```python
from build123d import *

# Parameters (mm, degrees)
BOSS_EXTRUDE1_DEPTH     = 76.2
SKETCH2_R               = 22.225
SKETCH2_R_2             = 4.7625
CUT_EXTRUDE2_DEPTH      = 34.20727615
CUT_EXTRUDE2_DEPTH_BACK = 31.29272385
CUT_EXTRUDE3_REACH      = 179.8
SKETCH3_R               = 6.35
SKETCH5_R               = 5.428392571
CUT_EXTRUDE4_DEPTH      = 76.2


with BuildPart() as part:
    # Sketch1 → Boss-Extrude1 (new body)
    with BuildSketch(Plane.XY):
        with BuildLine():
            Line((-88.9, -4.89272385), (73.025, -4.89272385))
            ThreePointArc((73.025, -4.89272385), (75.27006403, -5.82265982), (76.2, -8.06772385))
            Line((76.2, -8.06772385), (76.2, -30.29272385))
            Line((76.2, -30.29272385), (88.9, -30.29272385))
            Line((88.9, -30.29272385), (88.9, -4.89272385))
            Line((88.9, -4.89272385), (88.9, 7.80727615))
            Line((88.9, 7.80727615), (-73.025, 7.80727615))
            ThreePointArc((-73.025, 7.80727615), (-75.27006403, 8.73721212), (-76.2, 10.98227615))
            Line((-76.2, 10.98227615), (-76.2, 33.20727615))
            Line((-76.2, 33.20727615), (-88.9, 33.20727615))
            Line((-88.9, 33.20727615), (-88.9, 4.89272385))
            Line((-88.9, 4.89272385), (-88.9, -4.89272385))
        make_face()
    extrude(amount=BOSS_EXTRUDE1_DEPTH)

    # Sketch2 → Cut-Extrude2 (cut, two sides)
    with BuildSketch(Plane(origin=(0, 0, 0), x_dir=(1, 0, 0), z_dir=(0, 1, 0))) as cut_extrude2_sk:
        with Locations((0, -38.1)):
            Circle(SKETCH2_R)
        with Locations((-44.45, -38.1)):
            Circle(SKETCH2_R_2)
        with Locations((44.45, -38.1)):
            Circle(SKETCH2_R_2)
    extrude(amount=CUT_EXTRUDE2_DEPTH, mode=Mode.SUBTRACT)
    extrude(cut_extrude2_sk.sketch, amount=-CUT_EXTRUDE2_DEPTH_BACK, mode=Mode.SUBTRACT)

    # Sketch3 → Cut-Extrude3 (cut, up to next)
    with BuildSketch(Plane.ZY.offset(88.9), mode=Mode.PRIVATE) as cut_extrude3_sk1:
        with Locations((19.05, 20.50727615)):
            Circle(SKETCH3_R)
    cut_extrude3_tool1 = extrude(cut_extrude3_sk1.sketch, amount=-CUT_EXTRUDE3_REACH, mode=Mode.PRIVATE) & part.part
    add(cut_extrude3_tool1.solids().sort_by_distance((-88.9, 20.507276, 19.05))[0], mode=Mode.SUBTRACT)
    # Sketch3 → Cut-Extrude3 (cut, up to next)
    with BuildSketch(Plane.ZY.offset(88.9), mode=Mode.PRIVATE) as cut_extrude3_sk2:
        with Locations((57.15, 20.50727615)):
            Circle(SKETCH3_R)
    cut_extrude3_tool2 = extrude(cut_extrude3_sk2.sketch, amount=-CUT_EXTRUDE3_REACH, mode=Mode.PRIVATE) & part.part
    add(cut_extrude3_tool2.solids().sort_by_distance((-88.9, 20.507276, 57.15))[0], mode=Mode.SUBTRACT)

    # Sketch5 → Cut-Extrude4 (cut)
    with BuildSketch(Plane(origin=(88.9, 0, 0), x_dir=(0, 0, -1), z_dir=(1, 0, 0))):
        with Locations((-57.15, -17.59272385)):
            Circle(SKETCH5_R)
        with Locations((-19.05, -17.59272385)):
            Circle(SKETCH5_R)
    extrude(amount=-CUT_EXTRUDE4_DEPTH, mode=Mode.SUBTRACT)


solid = part.part
```
Input: part model. Units: mm. Frame: model coordinates. A direction names the side the tool comes from. Coordinates: 2 decimals unless noted, no trailing zeros. Write each loop counter-clockwise with the first axis right and the second up, starting at its lowest first coordinate (ties: lowest second). Pieces come first, ordered by that corner, then holes. Notation, with made-up numbers: M 44.25,-15.75 L 100.25,-15.75 A20 cw 100.25,0.25 Z; hole C 29.5,2 d2. An arc over 180 degrees is marked long. Use one line per item in the form item = value.
Q1. Material intervals for probe 1 along X at (y, z) = (-2, 38); probe 2 along X at (y, z) = (-11, 10); probe 3 along Y at (x, z) = (-49, 56), sorted ascending. Write a range as from..to.
Answer below:
probe_1 = -88.9..-49.21, -39.69..-22.22, 22.22..39.69, 49.21..88.9
probe_2 = 76.2..88.9
probe_3 = -4.89..7.81
Q2. Set-up query: faces 5 (the face through (82, -30.293, 38)), 6 (the face through (76.2, -19, 38)), 7 (the face through (27, 7.807, 38)). Return all of +Z, -Z, +X, -X, +Y, -Y with unobstructed straight access to the full face (end or side cutting, diameter ignored); none if empty.
Answer below:
face_5 = +Z, -Z, +X, -X, -Y
face_6 = +Z, -Z, -X, -Y
face_7 = +Z, -Z, +X, +Y
Q3. Draft query along Z for faces 1 (the face through (0, -1, 76.2)), 2 (the face through (0, -1, 0)), 3 (the face through (-75.245, 8.713, 37.567)), 4 (the face through (-82.639, 14.874, 21.98)). Return one class per face: released by +Z, released by -Z, zero draft, split by the parting line, or undercut.
Answer below:
face_1 = released by +Z
face_2 = released by -Z
face_3 = zero draft
face_4 = undercut
Q4. Section D-D (y = -26). Return loops of the section in (x, z), plus the area to 3 significant figures.
Answer below:
outline = M 76.2,0 L 88.9,0 L 88.9,76.2 L 76.2,76.2 Z
area = 968 mm²
Q5. Section C-C (x = 44.45). Return loops of the section in (y, z), plus the area to 3 significant figures.
Answer below:
outline = M -4.89,0 L 7.81,0 L 7.81,33.34 L -4.89,33.34 Z; M -4.89,42.86 L 7.81,42.86 L 7.81,76.2 L -4.89,76.2 Z
area = 847 mm²
Q6. Section A-A (z = 38.1). Count the separate pieces of the cut face and the enclosed holes in it, plus the area to 3 significant figures.
Answer below:
separate_pieces = 4
enclosed_holes = 0
area = 2,100 mm²
Q7. First-contact query: pin 1 (10 mm diameter, centred on y = 14.5, z = 17.5, fed in from +X); pin 2 (1.5 mm diameter, centred on x = -33.5, z = 60, fed in from -Y); pin 3 (11 mm diameter, centred on y = -15, z = 25, fed in from -X); pin 4 (10 mm diameter, centred on y = -17.59, z = 57.15, fed in from -X). Flat tips, straight axial feed; report the tip coordinate or a pass-through.
Answer below:
pin_1 = -75.83
pin_2 = -4.89
pin_3 = 76.2
pin_4 = through
Q8. Section B-B (x = 0). Return loops of the section in (y, z) (3 decimals).
Answer below:
outline = M -4.893,0 L 7.807,0 L 7.807,15.875 L -4.893,15.875 Z; M -4.893,60.325 L 7.807,60.325 L 7.807,76.2 L -4.893,76.2 Z
